Geometry check sheet. Reference: the model listing, model coordinates, mm. Face numbers are marked on the shaded views. Round coordinates to 2 decimals unless told otherwise and drop trailing zeros. Write each loop counter-clockwise with the first axis right and the second up, starting at its lowest first coordinate (ties: lowest second). Pieces come first, ordered by that corner, then holes. Notation, with made-up numbers: (-2.5, -26) -> (40.5, -26) arc R37 cw to (40.5, 13) -> close; hole circle Ø2 at (53.5, -28.5). An arc over 180 degrees is marked (long way). Use a Markdown table: item, result.
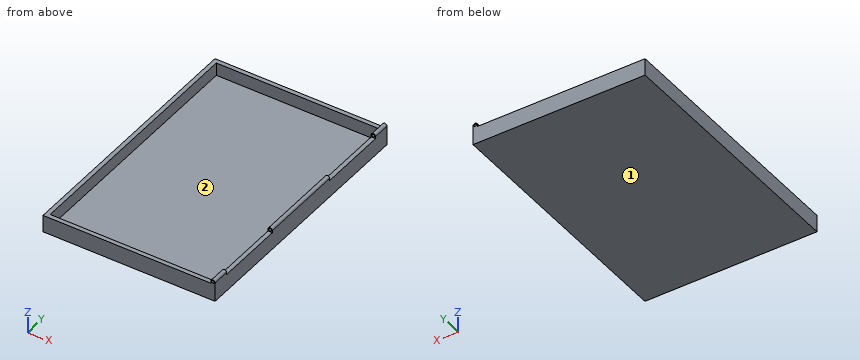
```python
from build123d import *

# Parameters (mm, degrees)
F0_W     = 254
F0_H     = 381
F0_W_2   = 241.3
F0_H_2   = 368.3
F1_DEPTH = 25.4
F2_DEPTH = 6.35
F4_START = -127
F3_R     = 1.905
F4_DEPTH = 127
F5_DEPTH = 25.4
F6_START = -355.6
F6_DEPTH = 25.4


with BuildPart() as f1:
    # F0 (on Top) → F1 (new body)
    with BuildSketch(Plane.XY):
        Rectangle(F0_W, F0_H)
        Rectangle(F0_W_2, F0_H_2, mode=Mode.SUBTRACT)
    extrude(amount=F1_DEPTH)

    # F0 (on Top) → F2 (join)
    with BuildSketch(Plane.XY):
        Rectangle(F0_W_2, F0_H_2)
    extrude(amount=F2_DEPTH)

    # F3 (on face) → F4 (join)
    with BuildSketch(Plane.XZ.offset(190.5).offset(F4_START)):
        with BuildLine():
            Line((120.65, 25.4), (127, 25.4))
            Line((127, 25.4), (127, 28.575))
            ThreePointArc((127, 28.575), (123.825, 31.75), (120.65, 28.575))
            Line((120.65, 28.575), (120.65, 25.4))
        make_face()
        with Locations((123.825, 28.575)):
            Circle(F3_R, mode=Mode.SUBTRACT)
    extrude(amount=-F4_DEPTH)

    # F3 (on face) → F5 (join)
    with BuildSketch(Plane.XZ.offset(190.5)):
        with BuildLine():
            Line((120.65, 25.4), (127, 25.4))
            Line((127, 25.4), (127, 28.575))
            ThreePointArc((127, 28.575), (123.825, 31.75), (120.65, 28.575))
            Line((120.65, 28.575), (120.65, 25.4))
        make_face()
        with Locations((123.825, 28.575)):
            Circle(F3_R, mode=Mode.SUBTRACT)
    extrude(amount=-F5_DEPTH)

    # F3 (on face) → F6 (join)
    with BuildSketch(Plane.XZ.offset(190.5).offset(F6_START)):
        with BuildLine():
            Line((120.65, 25.4), (127, 25.4))
            Line((127, 25.4), (127, 28.575))
            ThreePointArc((127, 28.575), (123.825, 31.75), (120.65, 28.575))
            Line((120.65, 28.575), (120.65, 25.4))
        make_face()
        with Locations((123.825, 28.575)):
            Circle(F3_R, mode=Mode.SUBTRACT)
    extrude(amount=-F6_DEPTH)


solid = f1.part
```
(1) Section check C-C on x = 49. Record the cut outline in (y, z), plus the area to 3 significant figures.
A:
| item | result |
|---|---|
| outline | (-190.5, 0) -> (190.5, 0) -> (190.5, 25.4) -> (184.15, 25.4) -> (184.15, 6.35) -> (-184.15, 6.35) -> (-184.15, 25.4) -> (-190.5, 25.4) -> close |
| area | 2,660 mm2 |
(2) Gauge pin test, flat ends, axial feed: pin 1 Ø5 at (x, y) = (124.5, -106.5) entering from +Z; pin 2 Ø3 at (x, z) = (123.825, 28.575) entering from -Y. Record the tip position at first contact, or that the pin passes through.
A:
| item | result |
|---|---|
| pin 1 | stops at z = 25.4 |
| pin 2 | passes through |
(3) Thickness scan on line 1 (X direction, y = -15, z = 14); line 2 (Y direction, x = 98.5, z = 16); line 3 (Z direction, x = 102, y = -21.5). Record the ranges inside material, lowest first.
A:
| item | result |
|---|---|
| line 1 | x = -127 to -120.65, 120.65 to 127 |
| line 2 | y = -190.5 to -184.15, 184.15 to 190.5 |
| line 3 | z = 0 to 6.35 |
(4) Section check B-B on y = -23. Record the cut outline in (x, z) (3 decimals), plus the area to 3 significant figures.
A:
| item | result |
|---|---|
| outline | (-127, 0) -> (127, 0) -> (127, 28.575) arc R3.175 ccw to (120.65, 28.575) -> (120.65, 6.35) -> (-120.65, 6.35) -> (-120.65, 25.4) -> (-127, 25.4) -> close; hole circle Ø3.81 at (123.825, 28.575) |
| area | 1,880 mm2 |
(5) Section check A-A on z = 11.5. Record the cut outline in (x, y).
A:
| item | result |
|---|---|
| outline | (-127, -190.5) -> (127, -190.5) -> (127, 190.5) -> (-127, 190.5) -> close; hole (-120.65, -184.15) -> (120.65, -184.15) -> (120.65, 184.15) -> (-120.65, 184.15) -> close |
(6) Section check D-D on y = -75. Record the cut outline in (x, z).
A:
| item | result |
|---|---|
| outline | (-127, 0) -> (127, 0) -> (127, 25.4) -> (120.65, 25.4) -> (120.65, 6.35) -> (-120.65, 6.35) -> (-120.65, 25.4) -> (-127, 25.4) -> close |
(7) Release check for a two-part mould opening along X. For the marked faces 1 and 2 record: +X half, -X half, draft (parallel to the pull), parting line (faces both ways), or undercut.
A:
| item | result |
|---|---|
| face 1 | draft |
| face 2 | undercut |
